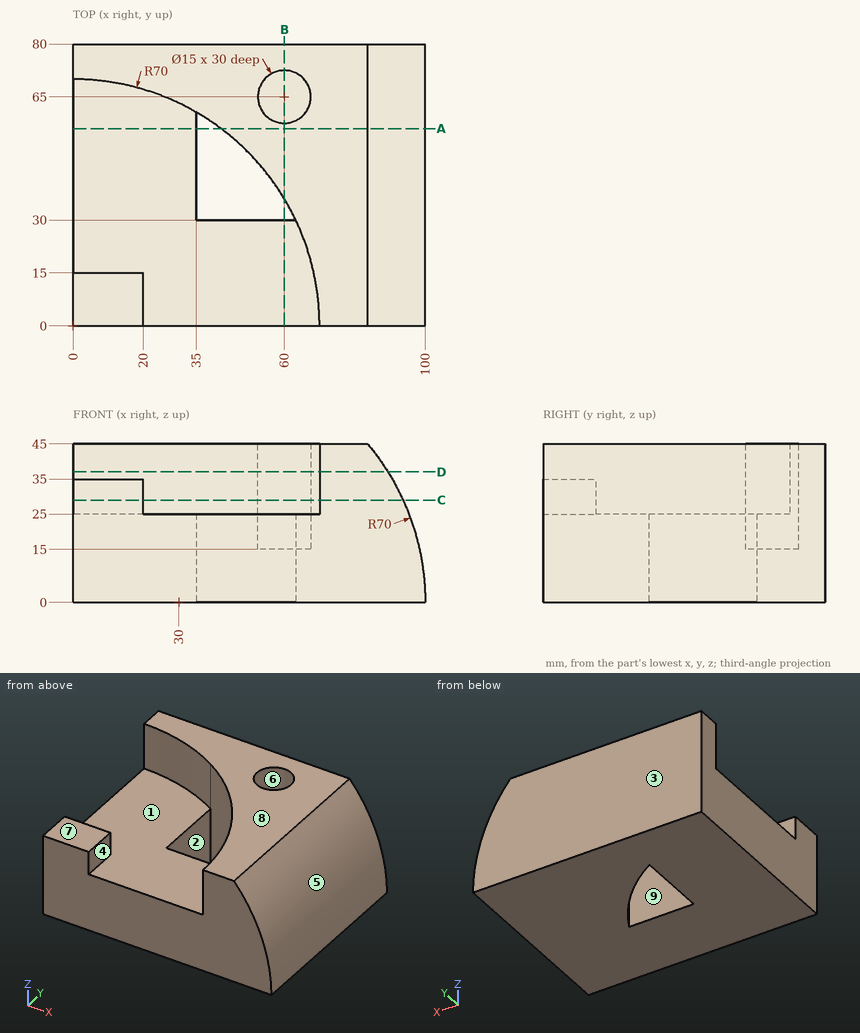
The drawing under review shows one solid part. Ordinate dimensions are in mm from its lowest x, y, z. A direction names the side the tool comes from. Coordinates: 2 decimals unless noted, no trailing zeros. Write each loop counter-clockwise with the first axis right and the second up, starting at its lowest first coordinate (ties: lowest second). Pieces come first, ordered by that corner, then holes.
1) Add section C-C (z = 29). Write out the cut boundary in (x, y), plus the area to 3 significant figures.
2) Insertion check: pin 1 (12 mm diameter, centred on y = 68.5, z = 12.5, fed in from +X); pin 2 (4.5 mm diameter, centred on x = 6.5, y = 8.5, fed in from +Z); pin 3 (5 mm diameter, centred on y = 4.5, z = 29, fed in from +X). Each pin has a flat end and moves straight along its axis. Give the tip position at first contact, or say it passes through.
3) Add section D-D (z = 37). Write out the cut boundary in (x, y), plus the area to 3 significant figures.
4) Machinability: for the marked faces 5, 6, 7, 8 and 9, which of the approach directions +Z, -Z, +X, -X, +Y, -Y give a long, thin tool a straight path to every point of the face, cutting with its end or side? Answer none if there is none.
5) Mouldability with a two-part tool opening along Y and no side actions: class the marked faces 1, 2, 3 and 4 as +Y half, -Y half, draft (parallel to the pull), parting line (faces both ways), or undercut.
6) Add section B-B (x = 60). Write out the cut boundary in (y, z), plus the area to 3 significant figures.
7) To check wall thickness, follow L1, parallel to Z at x = 20, y = 25; L2, parallel to Z at x = 19, y = 14.5; L3, parallel to X at y = 11.5, z = 27.5. State the ranges of each line that lie inside material, in increasing order.
8) Add section A-A (y = 56). Write out the cut boundary in (x, z).
Check result:
1. outline: (0, 0) - (20, 0) - (20, 15) - (0, 15) - close; (0, 70) arc R70 cw to (35, 60.62) arc R70 cw to (63.25, 30) arc R70 cw to (70, 0) - (93.71, 0) - (93.71, 80) - (0, 80) - close; hole circle Ø15 at (60, 65)
1. area: 3,770 mm2
2. pin 1: stops at x = 99.7
2. pin 2: stops at z = 35
2. pin 3: stops at x = 94.79
3. outline: (0, 70) arc R70 cw to (35, 60.62) arc R70 cw to (63.25, 30) arc R70 cw to (70, 0) - (89.42, 0) - (89.42, 80) - (0, 80) - close; hole circle Ø15 at (60, 65)
3. area: 3,130 mm2
4. face 5: +Z, +X, +Y, -Y
4. face 6: +Z
4. face 7: +Z, -X, -Y
4. face 8: +Z, +X, -X, +Y, -Y
4. face 9: +Z, -Z
5. face 1: undercut
5. face 2: undercut
5. face 3: +Y half
5. face 4: draft
6. outline: (0, 0) - (30, 0) - (30, 25) - (0, 25) - close; (36.06, 0) - (80, 0) - (80, 45) - (72.5, 45) - (72.5, 15) - (57.5, 15) - (57.5, 45) - (36.06, 45) - close
6. area: 2,280 mm2
7. L1: z = 0 to 25
7. L2: z = 0 to 35
7. L3: x = 0 to 20, 69.05 to 94.37
8. outline: (0, 0) - (35, 0) - (35, 25) - (0, 25) - close; (42, 0) - (100, 0) arc R70 ccw to (83.62, 45) - (42, 45) - close
